Could you check a few things on this model? Use its own coordinates, in mm. Face numbers are marked on the shaded views. Coordinates: 2 decimals unless noted, no trailing zeros. Loops run counter-clockwise (first coordinate to the right, second up) from the corner with the lowest first, then second, coordinate; pieces in that order, holes last. Notation, with made-up numbers: (-19.5, 64) - (-6.5, 64) arc R25 ccw to (-6.5, 92) - close; hole circle Ø1 at (-25.5, 63). An arc over 180 degrees is marked (long way). Use CSV: the item, a comma, the result in double quotes.
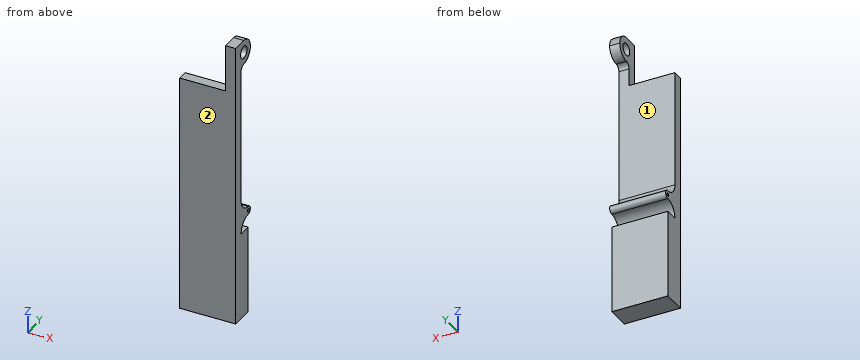
from build123d import *

# Parameters (mm, degrees)
SKETCH1_R           = 6
SKETCH1_R_2         = 1.5
BOSS_EXTRUDE1_DEPTH = 55
SKETCH2_W           = 45
SKETCH2_H           = 46
CUT_EXTRUDE1_DEPTH  = 290.556557515


with BuildPart() as part:
    # Sketch1 → Boss-Extrude1 (new body)
    with BuildSketch(Plane(origin=(0, 0, 0), x_dir=(0, 0, -1), z_dir=(1, 0, 0))):
        with BuildLine():
            Line((3, 15), (3, 0))
            Line((3, 0), (283, 0))
            Line((283, 0), (283, 23))
            Line((283, 23), (197, 23))
            Line((197, 23), (197, 10))
            ThreePointArc((197, 10), (187.807611845, 13.807611845), (184, 23))
            ThreePointArc((184, 23), (180, 27), (176, 23))
            ThreePointArc((176, 23), (172.192388155, 13.807611845), (163, 10))
            Line((163, 10), (32, 10))
            ThreePointArc((32, 10), (28.464466094, 11.464466094), (27, 15))
            ThreePointArc((27, 15), (23.485281374, 23.485281374), (15, 27))
            ThreePointArc((15, 27), (6.514718626, 23.485281374), (3, 15))
        make_face()
        with Locations((15, 15)):
            Circle(SKETCH1_R, mode=Mode.SUBTRACT)
        with Locations((180, 23)):
            Circle(SKETCH1_R_2, mode=Mode.SUBTRACT)
    extrude(amount=BOSS_EXTRUDE1_DEPTH)

    # Sketch2 → Cut-Extrude1 (cut, through all)
    with BuildSketch(Plane.XZ):
        with Locations((22.5, -26)):
            Rectangle(SKETCH2_W, SKETCH2_H)
    extrude(amount=-CUT_EXTRUDE1_DEPTH, mode=Mode.SUBTRACT)


solid = part.part
(1) Suppose I cut it at C-C (z = -230). Write out the boundary of the cut face in (x, y), plus the area to 4 significant figures.
Computed:
outline,"(0, 0) - (55, 0) - (55, 23) - (0, 23) - close"
area,"1,265 mm²"
(2) Suppose I cut it at B-B (z = -144). Write out the boundary of the cut face in (x, y), plus the area to 3 significant figures.
Computed:
outline,"(0, 0) - (55, 0) - (55, 10) - (0, 10) - close"
area,"550 mm²"
(3) Please list where these lines run through material, in increasing order: line 1 (Y direction, x = 13.5, z = -180); line 2 (Z direction, x = 52, y = 15); line 3 (Y direction, x = 51, z = -15).
Computed:
line 1,"y = 0 to 21.5, 24.5 to 27"
line 2,"z = -283 to -197, -186.75 to -173.25, -27 to -21, -9 to -3"
line 3,"y = 0 to 9, 21 to 27"
(4) Thinking about a two-plate mould opening in Z: for the marked faces 1 and 2, which applies, +Z half, -Z half, draft (parallel to the pull), parting line (faces both ways), or undercut?
Computed:
face 1,"undercut"
face 2,"draft"
(5) Suppose I cut it at A-A (x = 16.5). Write out the boundary of the cut face in (y, z), plus the area to 3 significant figures.
Computed:
outline,"(0, -283) - (23, -283) - (23, -197) - (10, -197) arc R13 cw to (23, -184) arc R4 ccw to (23, -176) arc R13 cw to (10, -163) - (10, -49) - (0, -49) - close; hole circle Ø3 at (23, -180)"
area,"3,650 mm²"
(6) Will these pins go through, and if not, where does the flat tip stop? pin 1 (11 mm diameter, centred on x = 24.5, y = 7, fed in from +Z); pin 2 (10 mm diameter, centred on y = 16.5, z = -36.5, fed in from +X); pin 3 (14 mm diameter, centred on y = 15, z = -15, fed in from -X); pin 4 (12 mm diameter, centred on x = 18.5, z = -206.5, fed in from +Y).
Computed:
pin 1,"stops at z = -49"
pin 2,"passes through"
pin 3,"stops at x = 45"
pin 4,"stops at y = 23"
